Here's how the part is built. I have some questions about the finished solid (model axes, mm). A direction names the side the tool comes from. Coordinates: 2 decimals unless noted, no trailing zeros. Write each loop counter-clockwise with the first axis right and the second up, starting at its lowest first coordinate (ties: lowest second). Pieces come first, ordered by that corner, then holes. Notation, with made-up numbers: (60, 17) -> (84, 17) arc R13 cw to (84, 32) -> close; hole circle Ø9 at (34, -5). An arc over 180 degrees is marked (long way). Use CSV: the item, a comma, the result in double quotes. Start each with the question number.
```python
from build123d import *

# Parameters (mm, degrees)
SKETCH2_W           = 25
SKETCH2_H           = 20
BOSS_EXTRUDE1_DEPTH = 20
CHAMFER1_SIZE       = 1.5
SKETCH3_R           = 6
BOSS_EXTRUDE2_DEPTH = 1.5


with BuildPart() as part:
    # Sketch2 → Boss-Extrude1 (new body)
    with BuildSketch(Plane.XY):
        Rectangle(SKETCH2_W, SKETCH2_H)
    extrude(amount=BOSS_EXTRUDE1_DEPTH)

    # Chamfer1
    chamfer1_edges = [part.edges().sort_by_distance(p)[0] for p in [
        (12.5, -10, 10),
        (-12.5, -10, 10),
        (-12.5, 10, 10),
        (12.5, 10, 10),
    ]]
    chamfer(chamfer1_edges, length=CHAMFER1_SIZE)

    # Sketch3 → Boss-Extrude2 (add)
    with BuildSketch(Plane.XY.offset(20)):
        Circle(SKETCH3_R)
    extrude(amount=BOSS_EXTRUDE2_DEPTH)


solid = part.part
```
Item 1: If I drill on line 1 along Z through (x, y) = (10, 1), over which ranges is the centre line in solid material (lowest first)?
Item 2: I want a section at A-A on y = 0. Please give me the cut outline in (x, z).
Item 3: I'm going to push a flat-ended pin straight in: pin 1 (1 mm diameter, centred on x = -3.5, y = -7.5, fed in from -Z). Where does the tip first touch, or does it pass through?
Item 4: I want a section at C-C on x = -9. Please give me the cut outline in (y, z).
Item 5: I want a section at B-B on x = 0. Please give me the cut outline in (y, z).
Item 6: Which directions (+Z, -Z, +X, -X, +Y, -Y) give clear straight access to the entire face, cutting with the end or side of a thin tool? Please do faces 1 (the flat face through (0, -10, 10)), 2 (the flat face through (-6, -2, 20)).
Geometry says:
1,line 1,"0 to 20"
2,outline,"(-12.5, 0) -> (12.5, 0) -> (12.5, 20) -> (6, 20) -> (6, 21.5) -> (-6, 21.5) -> (-6, 20) -> (-12.5, 20) -> close"
3,pin 1,"z = 0"
4,outline,"(-10, 0) -> (10, 0) -> (10, 20) -> (-10, 20) -> close"
5,outline,"(-10, 0) -> (10, 0) -> (10, 20) -> (6, 20) -> (6, 21.5) -> (-6, 21.5) -> (-6, 20) -> (-10, 20) -> close"
6,face 1,"+Z, -Z, +X, -X, -Y"
6,face 2,"+Z"
